from build123d import *

# Parameters (mm, degrees)
F0_W     = 660.4
F0_H     = 50.8
F1_DEPTH = 50.8
F2_W     = 50.8
F2_H     = 50.8
F2_W_2   = 25.4
F2_H_2   = 15.24
F3_DEPTH = 50.8
F5_DEPTH = 50.8


with BuildPart() as f1:
    # F0 (on Top) → F1 (new body)
    with BuildSketch(Plane.XY):
        Rectangle(F0_W, F0_H)
    extrude(amount=F1_DEPTH)

    # F2 (on face) → F3 (cut)
    with BuildSketch(Plane(origin=(-330.2, 0, 0), x_dir=(0, -1, 0), z_dir=(-1, 0, 0))):
        with Locations((0, 25.4)):
            Rectangle(F2_W, F2_H)
        with Locations((0, 25.4)):
            Rectangle(F2_W_2, F2_H_2, mode=Mode.SUBTRACT)
    extrude(amount=-F3_DEPTH, mode=Mode.SUBTRACT)

    # F4 (on face) → F5 (cut)
    with BuildSketch(Plane.YZ.offset(330.2)):
        Polygon((-12.7, 17.78), (-25.4, 17.78), (-25.4, 0), (0, 0), (25.4, 0), (25.4, 17.78), (12.7, 17.78), align=None)
        Polygon((-25.4, 33.02), (-25.4, 17.78), (-12.7, 17.78), (-12.7, 25.4), (-12.7, 33.02), align=None)
        Polygon((-25.4, 50.8), (-25.4, 33.02), (-12.7, 33.02), (12.7, 33.02), (25.4, 33.02), (25.4, 50.8), (0, 50.8), align=None)
        Polygon((12.7, 25.4), (12.7, 17.78), (25.4, 17.78), (25.4, 33.02), (12.7, 33.02), align=None)
    extrude(amount=-F5_DEPTH, mode=Mode.SUBTRACT)


solid = f1.part
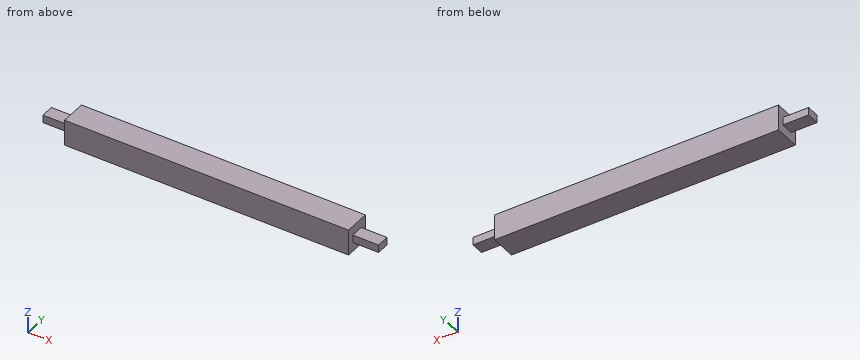
Can you work these out from the model? Positions are in its coordinate system, mm. Give positions to 0.01 mm unless a question says otherwise; leave off trailing zeros. Loops run counter-clockwise (first coordinate to the right, second up) from the corner with the lowest first, then second, coordinate; pieces in that order, holes last. Notation, with made-up numbers: (13, 63) -> (56, 63) arc R18 cw to (56, 84) -> close; hole circle Ø5 at (52.25, 40). An arc over 180 degrees is marked (long way). Write item = value, one per line.
1) Will these pins go through, and if not, where does the flat tip stop? pin 1 (20.5 mm diameter, centred on x = 292.5, y = 1, fed in from +Z); pin 2 (7.5 mm diameter, centred on x = -314.5, y = 5, fed in from -Z); pin 3 (17 mm diameter, centred on x = -298.5, z = 26.5, fed in from -Y); pin 4 (8 mm diameter, centred on y = 16.5, z = 19, fed in from +X).
Check result:
pin_1 = 33.02
pin_2 = 17.78
pin_3 = -12.7
pin_4 = 330.2
2) Suppose I cut it at A-A on y = 6. Write out the boundary of the cut face in (x, z).
Check result:
outline = (-330.2, 17.78) -> (-279.4, 17.78) -> (-279.4, 0) -> (279.4, 0) -> (279.4, 17.78) -> (330.2, 17.78) -> (330.2, 33.02) -> (279.4, 33.02) -> (279.4, 50.8) -> (-279.4, 50.8) -> (-279.4, 33.02) -> (-330.2, 33.02) -> close
3) I need wall thicknesses on L1, parallel to X at y = 18.5, z = 16; L2, parallel to Y at x = -287, z = 28. Which ranges of each line are inside material? Lowest first, please. Write a range as from..to.
Check result:
L1 = -279.4..279.4
L2 = -12.7..12.7
4) Suppose I cut it at B-B on z = 23.5. Write out the boundary of the cut face in (x, y).
Check result:
outline = (-330.2, -12.7) -> (-279.4, -12.7) -> (-279.4, -25.4) -> (279.4, -25.4) -> (279.4, -12.7) -> (330.2, -12.7) -> (330.2, 12.7) -> (279.4, 12.7) -> (279.4, 25.4) -> (-279.4, 25.4) -> (-279.4, 12.7) -> (-330.2, 12.7) -> close
